Geometry: see drawing. Coordinates: mm, zero at the bounding-box minimum. A direction names the side the tool comes from. Coordinates: 2 decimals unless noted, no trailing zeros. Loops run counter-clockwise (first coordinate to the right, second up) from the corner with the lowest first, then second, coordinate; pieces in that order, holes last. Notation, with made-up numbers: (-34, 79.5) -> (-11, 79.5) arc R13 cw to (-11, 101.5) -> close; hole circle Ø1 at (27, 64.5). An arc over 180 degrees is marked (long way). Answer as a JSON object with one key per item and string values.
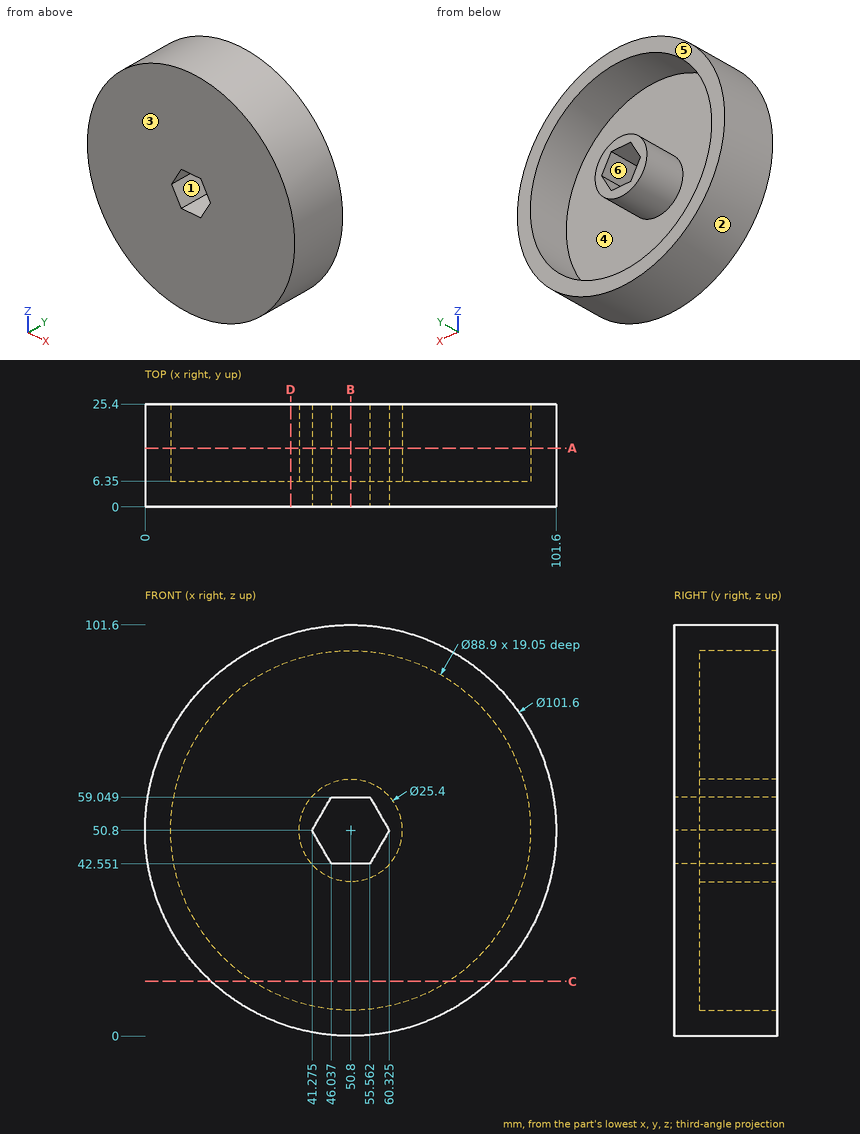
1. Section query A-A (y = 14.5). Count the separate pieces of the cut face and the enclosed holes in it, plus the area to 3 significant figures.
Reply:
{"separate pieces": "2", "enclosed holes": "2", "area": "2,170 mm2"}
2. Line query: line 1 along Y through (x, z) = (32, 76); line 2 along Z through (x, y) = (64, 17.75) (1 decimal); line 3 along X through (y, z) = (21.25, 89) (1 decimal). Output: solid intervals per line, ascending.
Reply:
{"line 1": "y = 0 to 6.35", "line 2": "z = 1.7 to 8.4, 93.2 to 99.9", "line 3": "x = 17.3 to 28.1, 73.5 to 84.3"}
3. Pin query (flat end, axial travel): P1, Ø8, axis at x = 73, z = 48.5, coming from the +Y side; P2, Ø8, axis at y = 13.5, z = 25, coming from the -X side (1 decimal); P3, Ø2, axis at x = 15, y = 9.5, coming from the -Z side. Return the tip coordinate at first contact, or that it passes through.
Reply:
{"P1": "stops at y = 6.35", "P2": "stops at x = 4.9", "P3": "stops at z = 13.79"}
4. Section query C-C (z = 13.5). Return loops of the section in (x, y).
Reply:
{"outline": "(16.31, 0) -> (85.29, 0) -> (85.29, 25.4) -> (74.98, 25.4) -> (74.98, 6.35) -> (26.62, 6.35) -> (26.62, 25.4) -> (16.31, 25.4) -> close"}
5. Section query B-B (x = 50.8). Return loops of the section in (y, z).
Reply:
{"outline": "(0, 0) -> (25.4, 0) -> (25.4, 6.35) -> (6.35, 6.35) -> (6.35, 38.1) -> (25.4, 38.1) -> (25.4, 42.55) -> (0, 42.55) -> close; (0, 59.05) -> (25.4, 59.05) -> (25.4, 63.5) -> (6.35, 63.5) -> (6.35, 95.25) -> (25.4, 95.25) -> (25.4, 101.6) -> (0, 101.6) -> close"}
6. Section query D-D (x = 36). Return loops of the section in (y, z).
Reply:
{"outline": "(0, 2.2) -> (25.4, 2.2) -> (25.4, 8.89) -> (6.35, 8.89) -> (6.35, 92.71) -> (25.4, 92.71) -> (25.4, 99.4) -> (0, 99.4) -> close"}
7. Mould query, pull axis X, two halves, no side actions, for the marked faces 1, 2 and 3. Classes: pulls with the +X half, pulls with the -X half, needs draft (parallel to the pull), parting line crosses it, or undercut.
Reply:
{"face 1": "undercut", "face 2": "parting line crosses it", "face 3": "needs draft"}
8. Access query for the marked faces 4, 5 and 6. Directions: +Z, -Z, +X, -X, +Y, -Y. A direction counts if a zero-diameter tool reaches every point of the face in a straight line with its end or side. Return the directions, or none.
Reply:
{"face 4": "+Y", "face 5": "+Z, -Z, +X, -X, +Y", "face 6": "+Y, -Y"}
